Source: CAD feature listing. Evaluate the final solid. Frame: model axes, mm. A direction names the side the tool comes from. Give positions to 0.01 mm unless a question says otherwise; leave off trailing zeros. Write each loop counter-clockwise with the first axis right and the second up, starting at its lowest first coordinate (ties: lowest second). Pieces come first, ordered by that corner, then holes. Notation, with made-up numbers: (43.5, 40) -> (63.5, 40) arc R27 ccw to (63.5, 75) -> close; hole circle Ø3 at (31, -36.75). An arc over 180 degrees is marked (long way). Use a Markdown table: item, result. Add a question column.
```python
from build123d import *

# Parameters (mm, degrees)
EXTRUDE_1_DEPTH          = 3.6
EXTRUDE_START            = -0.425
SKETCH_2_W               = 4.2
SKETCH_2_H               = 9
EXTRUDE_2_DEPTH          = 6.35
CUT_EXTRUDE_1_DEPTH      = 20.106543382
CUT_EXTRUDE_1_DEPTH_BACK = 20.106543382
SKETCH_2_3_R             = 1.6
SKETCH_5_W               = 13.4
SKETCH_5_H               = 11.925
EXTRUDE_3_DEPTH          = 6.2
SKETCH_6_R               = 2.3
EXTRUDE_4_DEPTH          = 2
CUT_EXTRUDE_2_DEPTH      = 29.741259541
CUT_EXTRUDE_2_DEPTH_BACK = 29.741259541


with BuildPart() as part:
    # Sketch 1 → Extrude 1 (new, symmetric)
    with BuildSketch(Plane.XY):
        with BuildLine():
            Line((-12.1, -3.6), (-6.7, -3.6))
            Line((-6.7, -3.6), (-6.7, -3.175))
            Line((-6.7, -3.175), (6.7, -3.175))
            Line((6.7, -3.175), (6.7, -3.6))
            Line((6.7, -3.6), (12.1, -3.6))
            ThreePointArc((12.1, -3.6), (12.807106781, -3.307106781), (13.1, -2.6))
            Line((13.1, -2.6), (13.1, 2.6))
            ThreePointArc((13.1, 2.6), (12.807106781, 3.307106781), (12.1, 3.6))
            Line((12.1, 3.6), (6.7, 3.6))
            Line((6.7, 3.6), (6.7, 3.175))
            Line((6.7, 3.175), (-6.7, 3.175))
            Line((-6.7, 3.175), (-6.7, 3.6))
            Line((-6.7, 3.6), (-12.1, 3.6))
            ThreePointArc((-12.1, 3.6), (-12.807106781, 3.307106781), (-13.1, 2.6))
            Line((-13.1, 2.6), (-13.1, -2.6))
            ThreePointArc((-13.1, -2.6), (-12.807106781, -3.307106781), (-12.1, -3.6))
        make_face()
        with BuildLine():
            Line((11.5, -1.6), (7.5, -1.6))
            ThreePointArc((7.5, -1.6), (7.112876483, 0), (7.5, 1.6))
            Line((7.5, 1.6), (11.5, 1.6))
            ThreePointArc((11.5, 1.6), (11.887123517, 0), (11.5, -1.6))
        make_face(mode=Mode.SUBTRACT)
        with BuildLine():
            Line((-11.5, 1.6), (-7.5, 1.6))
            ThreePointArc((-7.5, 1.6), (-7.112876483, 0), (-7.5, -1.6))
            Line((-7.5, -1.6), (-11.5, -1.6))
            ThreePointArc((-11.5, -1.6), (-11.887123517, 0), (-11.5, 1.6))
        make_face(mode=Mode.SUBTRACT)
    extrude(amount=EXTRUDE_1_DEPTH, both=True)

    # Sketch 2 → Extrude 2 (add)
    with BuildSketch(Plane(origin=(0, 3.6, 0), x_dir=(1, 0, 0), z_dir=(0, 1, 0)).offset(EXTRUDE_START)):
        with Locations((4.6, 7.4)):
            Rectangle(SKETCH_2_W, SKETCH_2_H)
        with Locations((-4.6, 7.4)):
            Rectangle(SKETCH_2_W, SKETCH_2_H)
    extrude(amount=-EXTRUDE_2_DEPTH)

    # Sketch 2_3 → Cut-Extrude 1 (cut, two sides: drawn at the far end of the back side and taken through both)
    with BuildSketch(Plane(origin=(0, 3.6, 0), x_dir=(1, 0, 0), z_dir=(0, 1, 0)).offset(-CUT_EXTRUDE_1_DEPTH_BACK)):
        with Locations(Location((-9.5, 0, 0), (0, 0, 270))):
            Circle(SKETCH_2_3_R)
        with Locations((9.5, 0)):
            Circle(SKETCH_2_3_R)
    extrude(amount=CUT_EXTRUDE_1_DEPTH + CUT_EXTRUDE_1_DEPTH_BACK, mode=Mode.SUBTRACT)

    # Sketch 5 → Extrude 3 (add)
    with BuildSketch(Plane.XY.offset(3.6)):
        with Locations((0, -9.1375)):
            Rectangle(SKETCH_5_W, SKETCH_5_H)
    extrude(amount=-EXTRUDE_3_DEPTH)

    # Sketch 6 → Extrude 4 (add)
    with BuildSketch(Plane.XZ.offset(15.1)):
        with Locations((0, 0.8)):
            Circle(SKETCH_6_R)
    extrude(amount=EXTRUDE_4_DEPTH)

    # Sketch 7 → Cut-Extrude 2 (cut, two sides: drawn at the far end of the back side and taken through both)
    with BuildSketch(Plane.ZY.offset(6.7).offset(-CUT_EXTRUDE_2_DEPTH_BACK)):
        with BuildLine():
            Line((-8.8, -0.8), (-9.2, -0.8))
            ThreePointArc((-9.2, -0.8), (-10, 0), (-9.2, 0.8))
            Line((-9.2, 0.8), (-8.8, 0.8))
            ThreePointArc((-8.8, 0.8), (-8, 0), (-8.8, -0.8))
        make_face()
    extrude(amount=CUT_EXTRUDE_2_DEPTH + CUT_EXTRUDE_2_DEPTH_BACK, mode=Mode.SUBTRACT)


solid = part.part
```
(1) Cut plane D-D on z = -4.25. Return the cut outline in (x, y) (3 decimals).
(2) Cut plane B-B on z = -2. Return the cut outline in (x, y) (3 decimals), then the cut area to 3 significant figures.
(3) Cut plane C-C on x = -9.5. Return the cut outline in (y, z).
(4) Cut plane A-A on y = 0. Return the cut outline in (x, z), then the cut area to 3 significant figures.
(5) Material intervals for L1, parallel to Z at x = 9.5, y = -2.15; L2, parallel to Z at x = 3.5, y = -6.25; L3, parallel to X at y = 1.25, z = -0.5, sorted ascending.
(6) Access query for faces 1 (the flat face through (0, 3.175, -2)), 2 (the flat face through (8, 1.6, 1)), 3 (the flat face through (2.5, 0, -7.7)), 4 (the flat face through (-9, -3.6, 2)), 5 (the flat face through (9, -3.6, 2)). Directions: +Z, -Z, +X, -X, +Y, -Y. A direction counts if a zero-diameter tool reaches every point of the face in a straight line with its end or side. Return the directions, or none.
(7) Mould query, pull axis Y, two halves, no side actions, for faces 6 (the flat face through (0, -9, -2.6)), 7 (the flat face through (-3, -3.175, -7)), 8 (the cylindrical face through (12.815, 3.299, 0.05)), 9 (the cylindrical face through (11.887, 0.023, 0.05)). Classes: +Y half, -Y half, draft (parallel to the pull), parting line (faces both ways), or undercut.
(8) First-contact query: pin 1 Ø1 at (x, z) = (0.5, 0.5) entering from +Y (3 decimals); pin 2 Ø2.5 at (x, z) = (-9.5, -1.5) entering from -Y; pin 3 Ø5 at (x, y) = (11.5, -0.5) entering from -Z. Flat tips, straight axial feed; report the tip coordinate or a pass-through.
Output:
| question | item | result |
|---|---|---|
| 1 | outline | (-6.7, -3.175) -> (-2.5, -3.175) -> (-2.5, 3.175) -> (-6.7, 3.175) -> close; (2.5, -3.175) -> (6.7, -3.175) -> (6.7, 3.175) -> (2.5, 3.175) -> close |
| 2 | outline | (-13.1, -2.6) arc R1 ccw to (-12.1, -3.6) -> (-6.7, -3.6) -> (-6.7, -15.1) -> (6.7, -15.1) -> (6.7, -3.6) -> (12.1, -3.6) arc R1 ccw to (13.1, -2.6) -> (13.1, 2.6) arc R1 ccw to (12.1, 3.6) -> (6.7, 3.6) -> (6.7, 3.175) -> (-6.7, 3.175) -> (-6.7, 3.6) -> (-12.1, 3.6) arc R1 ccw to (-13.1, 2.6) -> close; hole (-11.5, -1.6) -> (-7.5, -1.6) arc R3.5 ccw to (-7.5, 1.6) -> (-11.5, 1.6) arc R3.5 ccw to start; hole (7.5, -1.6) -> (11.5, -1.6) arc R3.5 ccw to (11.5, 1.6) -> (7.5, 1.6) arc R3.5 ccw to start |
| 2 | area | 307 mm^2 |
| 3 | outline | (-3.6, -3.6) -> (-1.6, -3.6) -> (-1.6, -1.6) -> (-3.6, -1.6) -> close; (-3.6, 1.6) -> (-1.6, 1.6) -> (-1.6, 3.6) -> (-3.6, 3.6) -> close; (1.6, -3.6) -> (3.6, -3.6) -> (3.6, -1.6) -> (1.6, -1.6) -> close; (1.6, 1.6) -> (3.6, 1.6) -> (3.6, 3.6) -> (1.6, 3.6) -> close |
| 4 | outline | (-13.1, -3.6) -> (-11.89, -3.6) -> (-11.89, 3.6) -> (-13.1, 3.6) -> close; (-7.11, -3.6) -> (-6.7, -3.6) -> (-6.7, -8) -> (-2.5, -8) -> (-2.5, -3.6) -> (2.5, -3.6) -> (2.5, -8) -> (6.7, -8) -> (6.7, -3.6) -> (7.11, -3.6) -> (7.11, 3.6) -> (-7.11, 3.6) -> close; (-6.7, -11.9) -> (-2.5, -11.9) -> (-2.5, -10) -> (-6.7, -10) -> close; (2.5, -11.9) -> (6.7, -11.9) -> (6.7, -10) -> (2.5, -10) -> close; (11.89, -3.6) -> (13.1, -3.6) -> (13.1, 3.6) -> (11.89, 3.6) -> close |
| 4 | area | 173 mm^2 |
| 5 | L1 | -3.6 to -1.6, 1.6 to 3.6 |
| 5 | L2 | -2.6 to 3.6 |
| 5 | L3 | -13.1 to -11.66, -7.34 to 7.34, 11.66 to 13.1 |
| 6 | face 1 | +Z, -Z, +Y |
| 6 | face 2 | +Z, -Z |
| 6 | face 3 | -Z, +Y, -Y |
| 6 | face 4 | +Z, -Z, -X, -Y |
| 6 | face 5 | +Z, -Z, +X, -Y |
| 7 | face 6 | draft |
| 7 | face 7 | -Y half |
| 7 | face 8 | +Y half |
| 7 | face 9 | undercut |
| 8 | pin 1 | y = 3.175 |
| 8 | pin 2 | y = -3.6 |
| 8 | pin 3 | z = -3.6 |
